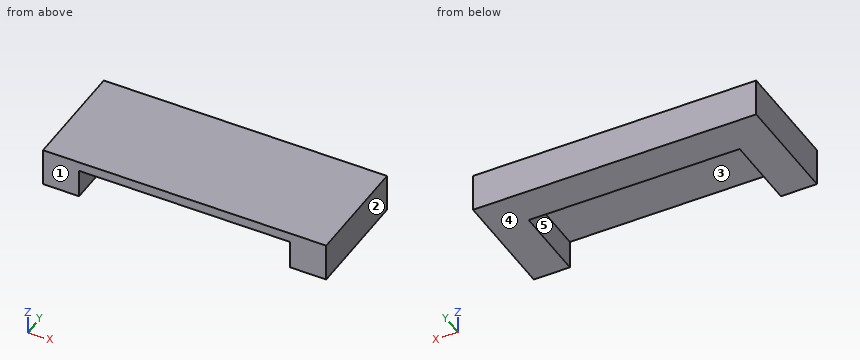
```python
from build123d import *

# Parameters (mm, degrees)
SKETCH001_W  = 11.1
SKETCH001_H  = 4
PAD001_DEPTH = 1.5
SKETCH_W     = 14.9
SKETCH_H     = 5.9
PAD_DEPTH    = 2


with BuildPart() as obj1:
    # Sketch001 → Pad001 (new body)
    with BuildSketch(Plane.XY):
        with Locations((0, -0.95)):
            Rectangle(SKETCH001_W, SKETCH001_H)
    extrude(amount=PAD001_DEPTH)


with BuildPart() as cut:
    # Sketch → Pad (new body)
    with BuildSketch(Plane.XY):
        Rectangle(SKETCH_W, SKETCH_H)
    extrude(amount=PAD_DEPTH)

    # Cut: cut obj1
    add(obj1.part, mode=Mode.SUBTRACT)


solid = cut.part
```
Verification items for the finished model (mm, model axes). Face numbers are marked on the shaded views. A direction names the side the tool comes from. Give positions to 0.01 mm unless a question says otherwise; leave off trailing zeros. Order: outer loops, then holes, each group sorted by start corner. A loop starts at its lowest first (then second) coordinate and runs counter-clockwise, first axis right, second up. Notation, with made-up numbers: (71, -33.5) - (82, -33.5) arc R28 ccw to (82, -2.5) - close; hole circle Ø6 at (-19.75, 47.5). An arc over 180 degrees is marked (long way). Answer as CSV lines item,"result". Start each with the question number.
Item 1: Section check A-A, the plane z = 1. Record the boundary of the cut face in (x, y).
Item 2: Material ranges on L1, parallel to X at y = -1.15, z = 1.15; L2, parallel to Y at x = 0.5, z = 0.45; L3, parallel to Z at x = 2.5, y = -1.9, recorded low to high.
Item 3: Mould release check, pull along X, two halves, no side actions. Record for the marked faces 1, 2 and 3: released by +X, released by -X, zero draft, split by the parting line, or undercut.
Item 4: Access from +Z, -Z, +X, -X, +Y, -Y to the whole of each face (thin tool, end or side, straight path). Record for the marked faces 4 and 5.
Item 5: Section check B-B, the plane y = 0.75. Record the boundary of the cut face in (x, z).
Item 6: Section check C-C, the plane x = 3.5. Record the boundary of the cut face in (y, z).
Item 7: Gauge pin test, flat ends, axial feed: pin 1 (0.8 mm diameter, centred on x = 1, z = 0.5, fed in from -Y); pin 2 (3 mm diameter, centred on x = -1.5, y = -1.5, fed in from -Z). Record the tip position at first contact, or that the pin passes through.
Filled in:
1,outline,"(-7.45, -2.95) - (-5.55, -2.95) - (-5.55, 1.05) - (5.55, 1.05) - (5.55, -2.95) - (7.45, -2.95) - (7.45, 2.95) - (-7.45, 2.95) - close"
2,L1,"-7.45 to -5.55, 5.55 to 7.45"
2,L2,"1.05 to 2.95"
2,L3,"1.5 to 2"
3,face 1,"zero draft"
3,face 2,"released by +X"
3,face 3,"undercut"
4,face 4,"-Z, +X, -X, +Y, -Y"
4,face 5,"-Z, -Y"
5,outline,"(-7.45, 0) - (-5.55, 0) - (-5.55, 1.5) - (5.55, 1.5) - (5.55, 0) - (7.45, 0) - (7.45, 2) - (-7.45, 2) - close"
6,outline,"(-2.95, 1.5) - (1.05, 1.5) - (1.05, 0) - (2.95, 0) - (2.95, 2) - (-2.95, 2) - close"
7,pin 1,"y = 1.05"
7,pin 2,"z = 1.5"
